Check sheet for the modelled part. Datum: model origin and axes. Units: mm. Coordinates: 2 decimals unless noted, no trailing zeros. Write each loop counter-clockwise with the first axis right and the second up, starting at its lowest first coordinate (ties: lowest second). Pieces come first, ordered by that corner, then holes. Notation, with made-up numbers: (-11, 37) - (9, 37) arc R28 cw to (9, 64) - close; hole circle Ø4 at (-33, -12). An arc over 180 degrees is marked (long way). Use one line per item in the form item = value. Start each with the question number.
1. Cross-section at A-A on x = 0. Record the boundary of the cut face in (y, z), then the cut area to 3 significant figures.
2. Scan lines: line 1 along Y through (x, z) = (-181.5, 2.1); line 2 along X through (y, z) = (-127, 1.7); line 3 along X through (y, z) = (-17, 1.8). Record each from-to range of solid material in increasing order.
3. Cross-section at C-C on z = 1.9. Give the number of separate pieces and of enclosed holes in the cut face, then the cut area to 3 significant figures.
4. Cross-section at B-B on y = 127. Record the boundary of the cut face in (x, z).
5. Cross-section at D-D on x = -45. Record the boundary of the cut face in (y, z), then the cut area to 3 significant figures.
6. Go/stop test with flat-tipped pins: pin 1 Ø11.5 at (x, y) = (182.372, 174.752) entering from -Z; pin 2 Ø2 at (x, y) = (-100, 1.5) entering from -Z. Record where each tip stops, or that it passes through.
7. Draft check along Y on faces 1 (the face through (-11.012, -104.194, 1.252)), 2 (the face through (-3, 3, 2.54)). Enter one of: +Y half, -Y half, draft (parallel to the pull), parting line (faces both ways), or undercut.
```python
from build123d import *

# Parameters (mm, degrees)
SKETCH_2_W          = 406.4
SKETCH_2_H          = 406.4
SKETCH_2_R          = 50.8
EXTRUDE_1_DEPTH     = 2.54
SKETCH_4_R          = 7.112
CUT_EXTRUDE_4_DEPTH = 288.379420975


with BuildPart() as part:
    # 草图2 → 凸台-拉伸1 (new body)
    with BuildSketch(Plane.XY):
        Rectangle(SKETCH_2_W, SKETCH_2_H)
        with Locations((0, -54.602000016)):
            Circle(SKETCH_2_R, mode=Mode.SUBTRACT)
    extrude(amount=EXTRUDE_1_DEPTH)

    # 草图4 → 切除-拉伸4 (cut, through all)
    with BuildSketch(Plane.XY):
        with Locations((-182.372, 127)):
            Circle(SKETCH_4_R)
        with Locations((-182.372, 174.752)):
            Circle(SKETCH_4_R)
        with Locations(Location((-182.372, -174.752, 0), (0, 0, 180))):
            Circle(SKETCH_4_R)
        with Locations(Location((-182.372, -127, 0), (0, 0, 180))):
            Circle(SKETCH_4_R)
        with Locations((182.372, -127)):
            Circle(SKETCH_4_R)
        with Locations((182.372, -174.752)):
            Circle(SKETCH_4_R)
        with Locations(Location((182.372, 174.752, 0), (0, 0, 180))):
            Circle(SKETCH_4_R)
        with Locations(Location((182.372, 127, 0), (0, 0, 180))):
            Circle(SKETCH_4_R)
    extrude(amount=CUT_EXTRUDE_4_DEPTH, mode=Mode.SUBTRACT)


solid = part.part
```
Final values:
q1.outline = (-203.2, 0) - (-105.4, 0) - (-105.4, 2.54) - (-203.2, 2.54) - close; (-3.8, 0) - (203.2, 0) - (203.2, 2.54) - (-3.8, 2.54) - close
q1.area = 774 mm²
q2.line_1 = -203.2 to -181.81, -167.69 to -134.06, -119.94 to 119.94, 134.06 to 167.69, 181.81 to 203.2
q2.line_2 = -203.2 to -189.48, -175.26 to 175.26, 189.48 to 203.2
q2.line_3 = -203.2 to -34.16, 34.16 to 203.2
q3.separate_pieces = 1
q3.enclosed_holes = 9
q3.area = 156,000 mm²
q4.outline = (-203.2, 0) - (-189.48, 0) - (-189.48, 2.54) - (-203.2, 2.54) - close; (-175.26, 0) - (175.26, 0) - (175.26, 2.54) - (-175.26, 2.54) - close; (189.48, 0) - (203.2, 0) - (203.2, 2.54) - (189.48, 2.54) - close
q5.outline = (-203.2, 0) - (-78.17, 0) - (-78.17, 2.54) - (-203.2, 2.54) - close; (-31.03, 0) - (203.2, 0) - (203.2, 2.54) - (-31.03, 2.54) - close
q5.area = 913 mm²
q6.pin_1 = through
q6.pin_2 = 0
q7.face_1 = undercut
q7.face_2 = draft
